```python
from build123d import *

# Parameters (mm, degrees)
ESQUISSE1_R        = 7.5
BOSS_EXTRU_1_DEPTH = 1
EXTRU_MINCE1_START = -3
EXTRU_MINCE1_DEPTH = 3
ESQUISSE2_W        = 4.681470229
ESQUISSE2_H        = 2.2


with BuildPart() as part:
    # Esquisse1 → Boss.-Extru.1 (new body)
    with BuildSketch(Plane.XY):
        Circle(ESQUISSE1_R)
    boss_extru_1 = extrude(amount=BOSS_EXTRU_1_DEPTH)

    # Esquisse1<3> → Extru.-Mince1 (add)
    with BuildSketch(Plane.XY.offset(EXTRU_MINCE1_START)):
        with BuildLine():
            ThreePointArc((0, 0.5), (0.28125, 0.413398642), (0.465073473, 0.18359375))
            Line((0.465073473, 0.18359375), (6.97610209, 2.75390625))
            ThreePointArc((6.97610209, 2.75390625), (4.21875, 6.200979635), (0, 7.5))
            Line((0, 7.5), (0, 0.5))
        make_face()
        with BuildLine():
            ThreePointArc((0.433012702, -0.25), (0.217388726, -0.450268966), (-0.073539885, -0.494562317))
            Line((-0.073539885, -0.494562317), (-1.103098273, -7.418434754))
            ThreePointArc((-1.103098273, -7.418434754), (3.260830893, -6.75403449), (6.495190528, -3.75))
            Line((6.495190528, -3.75), (0.433012702, -0.25))
        make_face()
        with BuildLine():
            ThreePointArc((-0.433012702, -0.25), (-0.498638726, 0.036870324), (-0.391533588, 0.310968567))
            Line((-0.391533588, 0.310968567), (-5.873003817, 4.664528504))
            ThreePointArc((-5.873003817, 4.664528504), (-7.479580893, 0.553054855), (-6.495190528, -3.75))
            Line((-6.495190528, -3.75), (-0.433012702, -0.25))
        make_face()
    extru_mince1 = extrude(amount=EXTRU_MINCE1_DEPTH)

    # Esquisse2 → Enlèvement de matière-Révolution1 (revolve, cut)
    with BuildSketch(Plane(origin=(0, 0, 0), x_dir=(1, 0, 0), z_dir=(0, 1, 0))):
        with Locations((-3.132268703, 1.5)):
            Rectangle(ESQUISSE2_W, ESQUISSE2_H)
    enl_vement_de_mati_re_r_volution1 = revolve(axis=Axis((-0.073539885, 0, -0.058266309), (0, 0, -1)), mode=Mode.SUBTRACT)

    # Symétrie1: Boss.-Extru.1, Extru.-Mince1, Enlèvement de matière-Révolution1 across plane
    add(boss_extru_1.mirror(Plane.XY.offset(1)))
    add(extru_mince1.mirror(Plane.XY.offset(1)))
    add(enl_vement_de_mati_re_r_volution1.mirror(Plane.XY.offset(1)), mode=Mode.SUBTRACT)


solid = part.part
```
Verification items for the finished model (mm, model axes). A direction names the side the tool comes from. Give positions to 0.01 mm unless a question says otherwise; leave off trailing zeros. Order: outer loops, then holes, each group sorted by start corner. A loop starts at its lowest first (then second) coordinate and runs counter-clockwise, first axis right, second up. Notation, with made-up numbers: (62, 37.5) - (114, 37.5) arc R22 cw to (114, 73.5) - close; hole circle Ø4 at (-21.5, 53.5). An arc over 180 degrees is marked (long way). Answer as CSV lines item,"result". Start each with the question number.
Item 1: Section check A-A, the plane y = 1.5. State how many separate pieces and enclosed holes the cut face has, plus the area to 3 significant figures.
Item 2: Access from +Z, -Z, +X, -X, +Y, -Y to the whole of each face (thin tool, end or side, straight path). Record for faces 1 (the face through (2, -4, -3)), 2 (the face through (-4, 0, 2.4)).
Item 3: Gauge pin test, flat ends, axial feed: pin 1 (1.5 mm diameter, centred on y = 5, z = -2, fed in from -X); pin 2 (1 mm diameter, centred on y = -2.5, z = 0, fed in from +X); pin 3 (2 mm diameter, centred on x = -2.5, y = -4, fed in from -Z). Record the tip position at first contact, or that the pin passes through.
Item 4: Mould release check, pull along X, two halves, no side actions. Record for faces 3 (the face through (-4, 0, -2.6)), 4 (the face through (4.85, -2.8, -1.52)), 5 (the face through (-5, 1, 5)): released by +X, released by -X, zero draft, split by the parting line, or undercut.
Item 5: Section check D-D, the plane x = 2.5. Record the boundary of the cut face in (y, z), plus the area to 3 significant figures.
Item 6: Section check B-B, the plane x = -2.75. Record the boundary of the cut face in (y, z), plus the area to 3 significant figures.
Item 7: Material ranges on L1, parallel to Z at x = 2, y = 3; L2, parallel to Z at x = -1, y = 5.25; L3, parallel to X at y = 3.25, z = 4, recorded low to high.
Item 8: Section check C-C, the plane z = 3.25. Record the boundary of the cut face in (x, y), plus the area to 3 significant figures.
Filled in:
1,separate pieces,"3"
1,enclosed holes,"0"
1,area,"53.4 mm^2"
2,face 1,"-Z, +X, -X, +Y, -Y"
2,face 2,"none"
3,pin 1,"x = -6.18"
3,pin 2,"x = 7.23"
3,pin 3,"z = 0"
4,face 3,"undercut"
4,face 4,"released by +X"
4,face 5,"zero draft"
5,outline,"(-7.07, -3) - (-1.44, -3) - (-1.44, -2.6) - (-4.75, -2.6) - (-4.75, -0.4) - (-1.44, -0.4) - (-1.44, 0) - (0.99, 0) - (0.99, -0.4) - (4.75, -0.4) - (4.75, -2.6) - (0.99, -2.6) - (0.99, -3) - (7.07, -3) - (7.07, 5) - (0.99, 5) - (0.99, 4.6) - (4.75, 4.6) - (4.75, 2.4) - (0.99, 2.4) - (0.99, 2) - (-1.44, 2) - (-1.44, 2.4) - (-4.75, 2.4) - (-4.75, 4.6) - (-1.44, 4.6) - (-1.44, 5) - (-7.07, 5) - close"
5,area,"67.5 mm^2"
6,outline,"(-6.98, 0) - (-1.59, 0) - (-1.59, -0.4) - (2.18, -0.4) - (2.18, 0) - (6.98, 0) - (6.98, 2) - (2.18, 2) - (2.18, 2.4) - (-1.59, 2.4) - (-1.59, 2) - (-6.98, 2) - close; (-1.59, -3) - (2.18, -3) - (2.18, -2.6) - (-1.59, -2.6) - close; (-1.59, 4.6) - (2.18, 4.6) - (2.18, 5) - (-1.59, 5) - close"
6,area,"33.9 mm^2"
7,L1,"-3 to -2.6, -0.4 to 2.4, 4.6 to 5"
7,L2,"0 to 2"
7,L3,"-6.76 to -4.39, 4.24 to 6.76"
8,outline,"(-6.5, -3.75) - (-4.73, -2.73) arc R5.4 cw to (-4.27, 3.39) - (-5.87, 4.66) arc R7.5 ccw to start; (-1.1, -7.42) arc R7.5 ccw to (6.5, -3.75) - (4.62, -2.67) arc R5.4 cw to (-0.8, -5.35) - close; (-0.68, -0.39) - (-0.43, -0.25) arc R0.5 cw to (-0.39, 0.31) - (-0.61, 0.48) arc R0.72 ccw to start; (-0.11, -0.72) arc R0.72 ccw to (0.57, -0.33) - (0.43, -0.25) arc R0.5 cw to (-0.07, -0.49) - close; (0, 0.5) arc R0.5 cw to (0.47, 0.18) - (0.6, 0.24) arc R0.72 ccw to (0, 0.71) - close; (0, 5.4) arc R5.4 cw to (4.96, 1.96) - (6.98, 2.75) arc R7.5 ccw to (0, 7.5) - close"
8,area,"49.0 mm^2"
